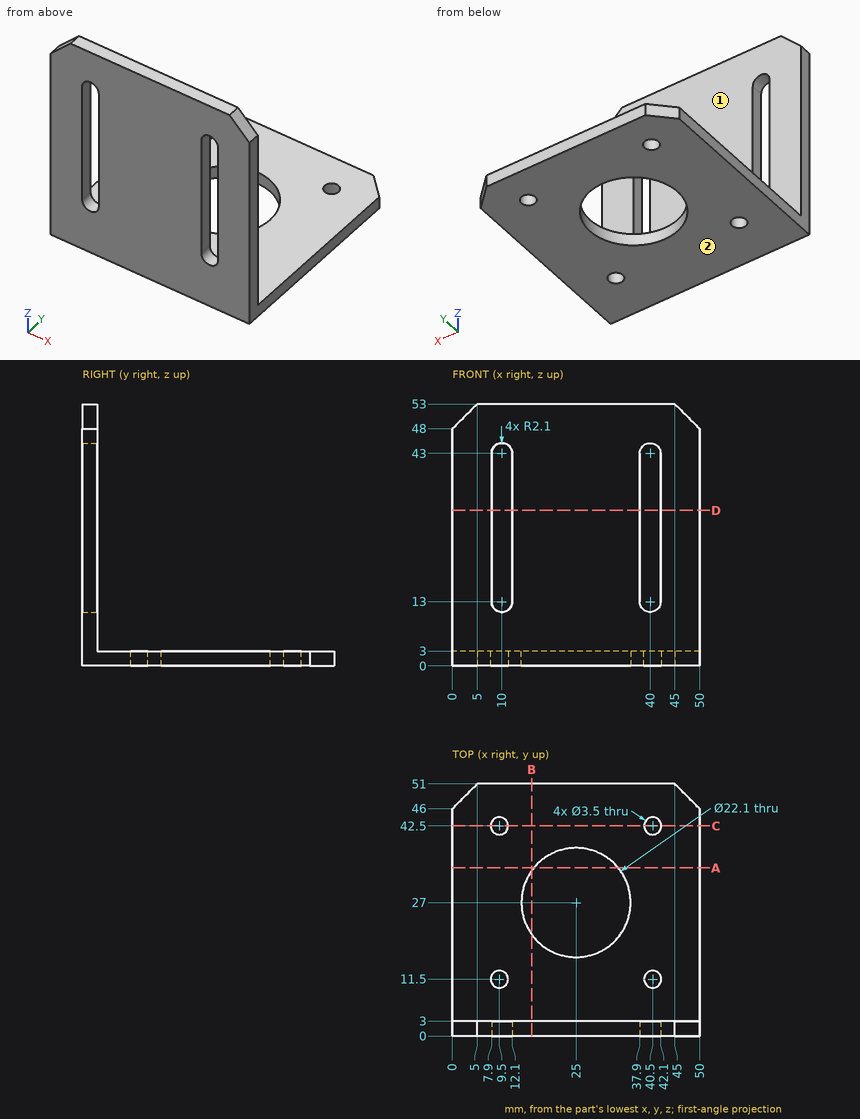
Geometry: see drawing. Coordinates: mm, zero at the bounding-box minimum. A direction names the side the tool comes from. Coordinates: 2 decimals unless noted, no trailing zeros. Loops run counter-clockwise (first coordinate to the right, second up) from the corner with the lowest first, then second, coordinate; pieces in that order, holes last.
Q1. Cut plane A-A (y = 34). Output: boundary loops of the cut face in (x, z), then the cut area to 3 significant figures.
Q2. Cut plane D-D (z = 31.5). Output: boundary loops of the cut face in (x, y), then the cut area to 3 significant figures.
Q3. Cut plane C-C (y = 42.5). Output: boundary loops of the cut face in (x, z), then the cut area to 3 significant figures.
Q4. Cut plane B-B (x = 16). Output: boundary loops of the cut face in (y, z), then the cut area to 3 significant figures.
Q5. Set-up query: the marked faces 1 and 2. Return all of +Z, -Z, +X, -X, +Y, -Y with unobstructed straight access to the full face (end or side cutting, diameter ignored); none if empty.
Q6. Material intervals for line 1 (Y direction, x = 9.5, z = 1.55); line 2 (Y direction, x = 25, z = 2); line 3 (X direction, y = 42, z = 1), sorted ascending.
Q7. Contact query for flat-ended pins moving along their axis: pin 1 (8 mm diameter, centred on x = 40.5, y = 20.5, fed in from +Z); pin 2 (2 mm diameter, centred on x = 44.5, z = 15, fed in from -Y); pin 3 (3 mm diameter, centred on x = 9.5, y = 42.5, fed in from +Z). Output: stop coordinate, or through.
Working result:
1. outline: (0, 0) - (16.45, 0) - (16.45, 3) - (0, 3) - close; (33.55, 0) - (50, 0) - (50, 3) - (33.55, 3) - close
1. area: 98.7 mm2
2. outline: (0, 0) - (7.9, 0) - (7.9, 3) - (0, 3) - close; (12.1, 0) - (37.9, 0) - (37.9, 3) - (12.1, 3) - close; (42.1, 0) - (50, 0) - (50, 3) - (42.1, 3) - close
2. area: 125 mm2
3. outline: (0, 0) - (7.75, 0) - (7.75, 3) - (0, 3) - close; (11.25, 0) - (38.75, 0) - (38.75, 3) - (11.25, 3) - close; (42.25, 0) - (50, 0) - (50, 3) - (42.25, 3) - close
3. area: 129 mm2
4. outline: (0, 0) - (20.59, 0) - (20.59, 3) - (3, 3) - (3, 53) - (0, 53) - close; (33.41, 0) - (51, 0) - (51, 3) - (33.41, 3) - close
4. area: 265 mm2
5. face 1: +Z, +X, -X, +Y
5. face 2: -Z, +X, -X, +Y, -Y
6. line 1: y = 0 to 9.75, 13.25 to 40.75, 44.25 to 51
6. line 2: y = 0 to 15.95, 38.05 to 51
6. line 3: x = 0 to 7.82, 11.18 to 38.82, 42.18 to 50
7. pin 1: stops at z = 3
7. pin 2: stops at y = 0
7. pin 3: passes through
